Could you check a few things on this model? Use its own coordinates, in mm. A direction names the side the tool comes from. Round coordinates to 2 decimals unless told otherwise and drop trailing zeros. Write each loop counter-clockwise with the first axis right and the second up, starting at its lowest first coordinate (ties: lowest second). Pieces come first, ordered by that corner, then holes. Notation, with made-up numbers: (20, 37) -> (50, 37) arc R16 cw to (50, 60) -> close; hole circle Ø7 at (71, 43). An arc over 180 degrees is marked (long way). One line per question, with ' | ' between items. Start each with the question number.
1. For faces 1 (the flat face through (-15, -0.4, -0.3)), 2 (the flat face through (3, -20, 0)), which set-ups out of +Z, -Z, +X, -X, +Y, -Y let a thin tool reach every point of the face, with its end or its side?
2. If I drill on line 1 along Z through (x, y) = (5, -17.15); line 2 along X through (y, z) = (1, 14.5); line 3 along Y through (x, z) = (-16.35, 0), over which ranges is the centre line in solid material (lowest first)? Write a range as [from, to].
3. Imagine slicing it at A-A, the plane z = 0. List the corners of the cut face in (x, y) for me, and give its area (3 significant figures).
4. For pin 1 Ø10 at (y, z) = (4.5, 2.5) entering from +X; pin 2 Ø16.5 at (x, z) = (11.5, 9.5) entering from +Y; pin 3 Ø10 at (x, z) = (-9.5, -8.5) entering from +Y; pin 4 Ø6 at (y, z) = (5, 0) entering from -X, each with a flat end and sliding along its axis, tell me the tip position at first contact or that it passes through.
5. Thinking about a two-plate mould opening in X: for faces 3 (the flat face through (-20, -0.4, 0.3)), 4 (the flat face through (20, -18, 0)), 5 (the cylindrical face through (3.85, -17.53, -12.22)), 6 (the flat face through (3, -15, 0)), which applies, released by +X, released by -X, zero draft, split by the parting line, or undercut?
6. Imagine slicing it at B-B, the plane y = 9. List the corners of the cut face in (x, z) for me.
7. Imagine slicing it at C-C, the plane x = 5. List the corners of the cut face in (y, z) for me, and give its area (3 significant figures).
8. Imagine slicing it at D-D, the plane z = -10. List the corners of the cut face in (x, y) for me.
from build123d import *

# Parameters (mm, degrees)
SKETCH1_W               = 40
SKETCH1_H               = 40
BOSS_EXTRUDE1_DEPTH     = 20
CUT_EXTRUDE1_DEPTH      = 49.989794856
CUT_EXTRUDE1_DEPTH_BACK = 49.989794856
SKETCH2_W               = 35
SKETCH2_H               = 35
FILLET1_R               = 2
FILLET2_R               = 7
HOLE1_D                 = 10
HOLE3_D                 = 5


with BuildPart() as part:
    # Sketch1 → Boss-Extrude1 (new, symmetric)
    with BuildSketch(Plane.XY):
        Rectangle(SKETCH1_W, SKETCH1_H)
    extrude(amount=BOSS_EXTRUDE1_DEPTH, both=True)

    # Sketch2 → Cut-Extrude1 (cut, two sides: drawn at the far end of the back side and taken through both)
    with BuildSketch(Plane.XY.offset(20).offset(-CUT_EXTRUDE1_DEPTH_BACK)):
        with Locations((2.5, 2.5)):
            Rectangle(SKETCH2_W, SKETCH2_H)
    extrude(amount=CUT_EXTRUDE1_DEPTH + CUT_EXTRUDE1_DEPTH_BACK, mode=Mode.SUBTRACT)

    # Fillet1
    fillet1_edges = [part.edges().sort_by_distance(p)[0] for p in [
        (-15, -15, 0),
    ]]
    fillet(fillet1_edges, radius=FILLET1_R)

    # Fillet2
    fillet2_edges = [part.edges().sort_by_distance(p)[0] for p in [
        (-20, -20, 0),
    ]]
    fillet(fillet2_edges, radius=FILLET2_R)

    # Hole1 (through all)
    with Locations(Plane(origin=(-15, 0, 0), x_dir=(0, 0, -1), z_dir=(1, 0, 0))):
        with Locations((0, 5)):
            Hole(HOLE1_D / 2)

    # Hole3 (through all)
    with Locations(Plane(origin=(0, -15, 0), x_dir=(1, 0, 0), z_dir=(0, 1, 0))):
        with Locations((5, -10)):
            hole3 = Hole(HOLE3_D / 2)

    # Mirror1: Hole3 across plane
    add(hole3.mirror(Plane.XY), mode=Mode.SUBTRACT)


solid = part.part
Geometry results:
1) face 1: +Z, -Z, +X, +Y | face 2: +Z, -Z, +X, -X, -Y
2) line 1: z = [-20, -12.5], [-7.5, 7.5], [12.5, 20] | line 2: x = [-20, -15] | line 3: y = [-19.15, 0], [10, 20]
3) outline: (-20, -13) arc R7 ccw to (-13, -20) -> (20, -20) -> (20, -15) -> (-13, -15) arc R2 cw to (-15, -13) -> (-15, 0) -> (-20, 0) -> close; (-20, 10) -> (-15, 10) -> (-15, 20) -> (-20, 20) -> close | area: 315 mm2
4) pin 1: stops at x = -15 | pin 2: stops at y = -15 | pin 3: stops at y = -14.32 | pin 4: passes through
5) face 3: released by -X | face 4: released by +X | face 5: undercut | face 6: zero draft
6) outline: (-20, -20) -> (-15, -20) -> (-15, -3) -> (-20, -3) -> close; (-20, 3) -> (-15, 3) -> (-15, 20) -> (-20, 20) -> close
7) outline: (-20, -20) -> (-15, -20) -> (-15, -12.5) -> (-20, -12.5) -> close; (-20, -7.5) -> (-15, -7.5) -> (-15, 7.5) -> (-20, 7.5) -> close; (-20, 12.5) -> (-15, 12.5) -> (-15, 20) -> (-20, 20) -> close | area: 150 mm2
8) outline: (-20, -13) arc R7 ccw to (-13, -20) -> (2.5, -20) -> (2.5, -15) -> (-13, -15) arc R2 cw to (-15, -13) -> (-15, 20) -> (-20, 20) -> close; (7.5, -20) -> (20, -20) -> (20, -15) -> (7.5, -15) -> close
